Autodesk Inventor part; units mm, degrees
ref_plane "YZ Plane" through (0, 0, 0) normal (1, 0, 0) x (0, 1, 0)
ref_plane "XZ Plane" through (0, 0, 0) normal (0, 1, 0) x (-1, 0, 0)
ref_plane "XY Plane" through (0, 0, 0) normal (0, 0, 1) x (1, 0, 0)
ref_plane "Arbeitsebene1" through (0, 0, 0) normal (0, 0, 1) x (1, 0, 0)
sketch "Skizze1" plane through (0, 0, 0) normal (0, 0, 1) x (1, 0, 0)
  circle A0 centre (-12, 2.9) radius 1.5
  circle A1 centre (12, 2.9) radius 1.5
  line L0 (-38, 12.9) -> (38, 12.9)
  line L1 (-38, -12.9) -> (-38, 12.9)
  line L2 (38, -12.9) -> (-38, -12.9)
  line L3 (38, 12.9) -> (38, -12.9)
  circle A2 centre (12, 2.9) radius 2.175
  circle A3 centre (-12, 2.9) radius 2.15
  circle A4 centre (-12, 2.9) radius 1.5
  circle A5 centre (12, 2.9) radius 1.5
  line L4 (-38, 12.9) -> (38, 12.9)
  line L5 (-38, -12.9) -> (-38, 12.9)
  line L6 (38, -12.9) -> (-38, -12.9)
  line L7 (38, 12.9) -> (38, -12.9)
  circle A6 centre (29, -0.15) radius 1.6
  circle A7 centre (-29, -0.15) radius 1.6
  circle A8 centre (29, -0.15) radius 2
  circle A9 centre (-29, -0.15) radius 2
  point P0 (0, 0)
  dimension "d0" = 4.35
  dimension "d1" = 4.3
  dimension "d2" = 4
  dimension "d3" = 4
extrude "Extrusion1" add sketch "Skizze1" along normal blind 5 contours L0 L3 L2 L1
properties part number "00_Sandwich_base"
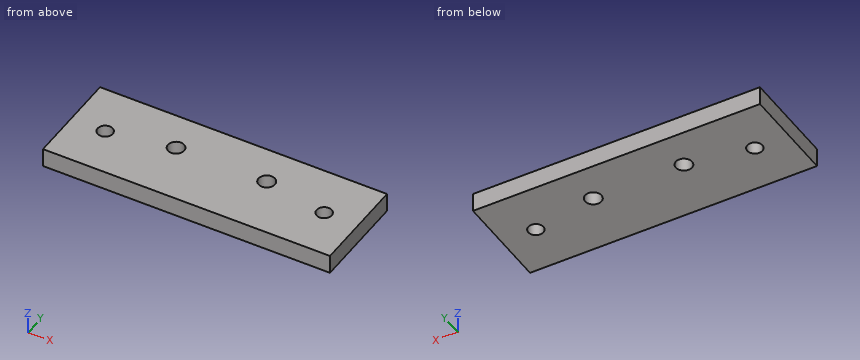
Source: CAD feature listing. Evaluate the final solid. Frame: model axes, mm. Coordinates: 2 decimals unless noted, no trailing zeros. Order: outer loops, then holes, each group sorted by start corner. A loop starts at its lowest first (then second) coordinate and runs counter-clockwise, first axis right, second up. Notation, with made-up numbers: (-38, 10.25) - (16, 10.25) arc R23 cw to (16, 34.25) - close; hole circle Ø8 at (53, 14). An arc over 180 degrees is marked (long way). One line per item, written item: value.
1) Cut plane D-D on x = 29. Output: boundary loops of the cut face in (y, z), plus the area to 3 significant figures.
Computed values:
outline: (-12.9, 0) - (-2.15, 0) - (-2.15, 5) - (-12.9, 5) - close; (1.85, 0) - (12.9, 0) - (12.9, 5) - (1.85, 5) - close
area: 109 mm^2
2) Cut plane B-B on z = 2.75. Output: boundary loops of the cut face in (x, y) (3 decimals).
Computed values:
outline: (-38, -12.9) - (38, -12.9) - (38, 12.9) - (-38, 12.9) - close; hole circle Ø4 at (-29, -0.15); hole circle Ø4.3 at (-12, 2.9); hole circle Ø4.35 at (12, 2.9); hole circle Ø4 at (29, -0.15)
3) Contact query for a flat-ended pin moving along its axis: pin 1 (5.5 mm diameter, centred on x = 12, y = 2.9, fed in from +Z). Output: stop coordinate, or through.
Computed values:
pin 1: stops at z = 5
4) Cut plane A-A on x = 12. Output: boundary loops of the cut face in (y, z) (3 decimals), plus the area to 3 significant figures.
Computed values:
outline: (-12.9, 0) - (0.725, 0) - (0.725, 5) - (-12.9, 5) - close; (5.075, 0) - (12.9, 0) - (12.9, 5) - (5.075, 5) - close
area: 107 mm^2
5) Cut plane C-C on y = 2.9. Output: boundary loops of the cut face in (x, z) (3 decimals), plus the area to 3 significant figures.
Computed values:
outline: (-38, 0) - (-14.15, 0) - (-14.15, 5) - (-38, 5) - close; (-9.85, 0) - (9.825, 0) - (9.825, 5) - (-9.85, 5) - close; (14.175, 0) - (38, 0) - (38, 5) - (14.175, 5) - close
area: 337 mm^2
6) Ray query, line 1 (Y direction, x = -29, z = 1.55); line 2 (X direction, y = 4.5, z = 3.1); line 3 (X direction, y = 1.5, z = 3.55). Return the intervals inside material, ascending. Write a range as [from, to].
Computed values:
line 1: y = [-12.9, -2.15], [1.85, 12.9]
line 2: x = [-38, -13.44], [-10.56, 10.53], [13.47, 38]
line 3: x = [-38, -30.13], [-27.87, -13.63], [-10.37, 10.34], [13.66, 27.87], [30.13, 38]
